from build123d import *

# Parameters (mm, degrees)
SKETCH_2_R                     = 12
EXTRUDE_2_DEPTH                = 12.4
SKETCH_5_R                     = 3.2
EXTRUDE_4_DEPTH                = 1
SKETCH_3_R                     = 1
EXTRUDE_3_DEPTH                = 8.6
SKETCH_6_R                     = 3
EXTRUDE_5_DEPTH                = 0.7
HOLE_WIZARD_M1_6_1_D           = 1.25
HOLE_WIZARD_M1_6_1_DEPTH       = 2
HOLE_WIZARD_M1_6_1_CSINK_D     = 1.3
HOLE_WIZARD_M1_6_1_CSINK_ANGLE = 90
HOLE_WIZARD_M1_6_1_TIP         = 0.375537887


with BuildPart() as part:
    # 草圖2 → 填料-伸長2 (new body)
    with BuildSketch(Plane(origin=(0, 0, 0), x_dir=(-1, 0, 0), z_dir=(0, 0, -1))):
        with Locations(Location((0, 0, 0), (0, 0, 180))):
            Circle(SKETCH_2_R)
    extrude(amount=EXTRUDE_2_DEPTH)

    # 草圖5 → 填料-伸長4 (add)
    with BuildSketch(Plane.XY):
        Circle(SKETCH_5_R)
    extrude(amount=EXTRUDE_4_DEPTH)

    # 草圖3 → 填料-伸長3 (add)
    with BuildSketch(Plane.XY.offset(1)):
        with Locations(Location((0, 0, 0), (0, 0, 180))):
            Circle(SKETCH_3_R)
    extrude(amount=EXTRUDE_3_DEPTH)

    # 草圖6 → 填料-伸長5 (add)
    with BuildSketch(Plane(origin=(0, 0, -12.4), x_dir=(-1, 0, 0), z_dir=(0, 0, -1))):
        Circle(SKETCH_6_R)
    extrude(amount=EXTRUDE_5_DEPTH)

    # M1.6  螺絲攻的螺孔鑽1
    with Locations(Plane.XY):
        with Locations((0, 8.25), (7.144709581, 4.125), (7.144709581, -4.125), (0, -8.25), (-7.144709581, -4.125), (-7.144709581, 4.125)):
            CounterSinkHole(HOLE_WIZARD_M1_6_1_D / 2, HOLE_WIZARD_M1_6_1_CSINK_D / 2, depth=HOLE_WIZARD_M1_6_1_DEPTH, counter_sink_angle=HOLE_WIZARD_M1_6_1_CSINK_ANGLE)
            with Locations((0, 0, -(HOLE_WIZARD_M1_6_1_DEPTH + HOLE_WIZARD_M1_6_1_TIP / 2))):  # 118° drill point
                Cone(0, HOLE_WIZARD_M1_6_1_D / 2, HOLE_WIZARD_M1_6_1_TIP, mode=Mode.SUBTRACT)


solid = part.part
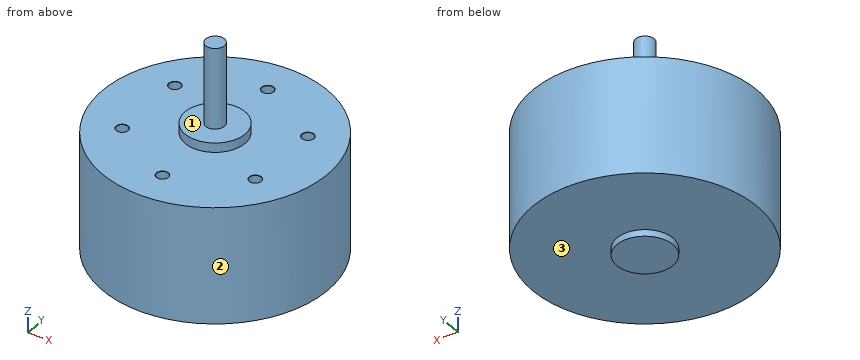
Verification items for the finished model (mm, model axes). Face numbers are marked on the shaded views. A direction names the side the tool comes from. Give positions to 0.01 mm unless a question says otherwise; leave off trailing zeros. Write each loop counter-clockwise with the first axis right and the second up, starting at its lowest first coordinate (ties: lowest second). Pieces come first, ordered by that corner, then holes. Notation, with made-up numbers: M 81,77 L 120,77 A24 cw 120,111 Z; hole C -31.75,-34.5 d5. An arc over 180 degrees is marked long. Use CSV: the item, a comma, the result in double quotes.
1) Access from +Z, -Z, +X, -X, +Y, -Y to the whole of each face (thin tool, end or side, straight path). Record for the marked faces 1, 2 and 3.
Final values:
face 1,"+Z"
face 2,"+Z, -Z"
face 3,"-Z"
2) Go/stop test with flat-tipped pins: pin 1 Ø1 at (x, y) = (0, -8.25) entering from +Z; pin 2 Ø8 at (x, y) = (-9, 4) entering from +Z; pin 3 Ø1 at (x, y) = (0, 8.25) entering from -Z. Record where each tip stops, or that it passes through.
Final values:
pin 1,"z = -2.08"
pin 2,"z = 0"
pin 3,"z = -12.4"
3) Cross-section at B-B (x = 1.5). Enter the section's corners in (y, z), plus the area to 3 significant figures.
Final values:
outline,"M -11.91,-12.4 L -2.6,-12.4 L -2.6,-13.1 L 2.6,-13.1 L 2.6,-12.4 L 11.91,-12.4 L 11.91,0 L 2.83,0 L 2.83,1 L -2.83,1 L -2.83,0 L -11.91,0 Z"
area,"305 mm²"
4) Cross-section at D-D (z = -11.25). Enter the section's corners in (x, y), plus the area to 3 significant figures.
Final values:
outline,"C 0,0 d24"
area,"452 mm²"
5) Material ranges on line 1 along Y through (x, z) = (0, -1.5) (3 decimals); line 2 along Z through (x, y) = (-3.75, 9.25); line 3 along X through (y, z) = (-8.25, -0.55) (3 decimals), recorded low to high.
Final values:
line 1,"-12 to -8.875, -7.625 to 7.625, 8.875 to 12"
line 2,"-12.4 to 0"
line 3,"-8.714 to -0.625, 0.625 to 8.714"
6) Cross-section at A-A (y = 0). Enter the section's corners in (x, z).
Final values:
outline,"M -12,-12.4 L -3,-12.4 L -3,-13.1 L 3,-13.1 L 3,-12.4 L 12,-12.4 L 12,0 L 3.2,0 L 3.2,1 L 1,1 L 1,9.6 L -1,9.6 L -1,1 L -3.2,1 L -3.2,0 L -12,0 Z"
7) Cross-section at C-C (z = 4.5). Enter the section's corners in (x, y).
Final values:
outline,"C 0,0 d2"
